```python
from build123d import *

# Parameters (mm, degrees)
BOSS_EXTRUDE1_DEPTH = 6.5
SKETCH2_W           = 15
SKETCH2_H           = 4
CUT_EXTRUDE1_DEPTH  = 3.5


with BuildPart() as part:
    # Sketch1 → Boss-Extrude1 (new body)
    with BuildSketch(Plane.XY):
        Polygon((0, 0), (-1.5, 1.5), (0, 1.5), (0, 5.5), (15, 5.5), (15, 1.5), (16.5, 1.5), (15, 0), align=None)
    extrude(amount=BOSS_EXTRUDE1_DEPTH)

    # Sketch2 → Cut-Extrude1 (cut)
    with BuildSketch(Plane.XY.offset(6.5)):
        with Locations((7.5, 3.5)):
            Rectangle(SKETCH2_W, SKETCH2_H)
    extrude(amount=-CUT_EXTRUDE1_DEPTH, mode=Mode.SUBTRACT)


solid = part.part
```
The model under review builds one solid part; all positions refer to its coordinate system, in mm. A direction names the side the tool comes from. Round coordinates to 2 decimals unless told otherwise and drop trailing zeros. Write each loop counter-clockwise with the first axis right and the second up, starting at its lowest first coordinate (ties: lowest second). Pieces come first, ordered by that corner, then holes. Notation, with made-up numbers: (68.5, 44.5) - (97.5, 44.5) arc R23 ccw to (97.5, 74.5) - close; hole circle Ø3 at (-11, -20.75). An arc over 180 degrees is marked (long way). One line per question, with ' | ' between items.
Item 1: For faces 1 (the face through (0, 3, 1)), 2 (the face through (7, 4, 3)), 3 (the face through (15, 4, 1)), 4 (the face through (8, 1, 6.5)), list the 3-axis set-ups (+Z, -Z, +X, -X, +Y, -Y) from which the entire face can be reached by the end or side of a thin tool; tool diameter is ignored.
Resolved:
face 1: +Z, -Z, -X, +Y | face 2: +Z, +X, -X, +Y | face 3: +Z, -Z, +X, +Y | face 4: +Z, +X, -X, +Y, -Y
Item 2: Add section C-C, the plane y = 0.65. Give the boundary of the cut face in (x, z), then the cut area to 3 significant figures.
Resolved:
outline: (-0.65, 0) - (15.65, 0) - (15.65, 6.5) - (-0.65, 6.5) - close | area: 106 mm2
Item 3: For P1, Ø3, axis at x = 11, y = 3.5, coming from the +Z side; P2, Ø1.5, axis at y = 4, z = 2, coming from the +X side; P3, Ø1.5, axis at x = 12.5, y = 4, coming from the -Z side; P4, Ø1.5, axis at y = 3.5, z = 5.5, coming from the +X side, all flat-tipped, find the tip position at first contact; note any pin that passes through.
Resolved:
P1: stops at z = 3 | P2: stops at x = 15 | P3: stops at z = 0 | P4: passes through
Item 4: Add section A-A, the plane z = 2.25. Give the boundary of the cut face in (x, y), then the cut area to 4 significant figures.
Resolved:
outline: (-1.5, 1.5) - (0, 0) - (15, 0) - (16.5, 1.5) - (15, 1.5) - (15, 5.5) - (0, 5.5) - (0, 1.5) - close | area: 84.75 mm2
Item 5: Add section B-B, the plane x = 11.5. Give the boundary of the cut face in (y, z).
Resolved:
outline: (0, 0) - (5.5, 0) - (5.5, 3) - (1.5, 3) - (1.5, 6.5) - (0, 6.5) - close
Item 6: To check wall thickness, follow probe 1 along Z at (x, y) = (2, 2.05); probe 2 along Y at (x, z) = (7.25, 4.75); probe 3 along X at (y, z) = (5.2, 1.75). State the ranges of each line that lie inside material, in increasing order.
Resolved:
probe 1: z = 0 to 3 | probe 2: y = 0 to 1.5 | probe 3: x = 0 to 15
Item 7: Add section D-D, the plane z = 5.75. Give the boundary of the cut face in (x, y), then the cut area to 4 significant figures.
Resolved:
outline: (-1.5, 1.5) - (0, 0) - (15, 0) - (16.5, 1.5) - close | area: 24.75 mm2
